```python
from build123d import *

# Parameters (mm, degrees)
SKETCH081_W      = 75
SKETCH081_H      = 95.5
EXTRUDE073_DEPTH = 1
SKETCH071_W      = 85
SKETCH071_H      = 109.5
EXTRUDE061_DEPTH = 2


with BuildPart() as extrude073:
    # Sketch081 → Extrude073 (new body)
    with BuildSketch(Plane.XY.offset(4)):
        with Locations((37.5, 49.25)):
            Rectangle(SKETCH081_W, SKETCH081_H)
    extrude(amount=EXTRUDE073_DEPTH)


with BuildPart() as cut008:
    # Sketch071 → Extrude061 (new body)
    with BuildSketch(Plane.XY.offset(3)):
        with Locations((37.5, 51.25)):
            Rectangle(SKETCH071_W, SKETCH071_H)
    extrude(amount=EXTRUDE061_DEPTH)

    # Cut008: cut Extrude073
    add(extrude073.part, mode=Mode.SUBTRACT)


solid = cut008.part
```
Geometry: final body of the model. Coordinates: model frame, mm. Coordinates: 2 decimals unless noted, no trailing zeros. Order: outer loops, then holes, each group sorted by start corner. A loop starts at its lowest first (then second) coordinate and runs counter-clockwise, first axis right, second up. Notation, with made-up numbers: (65.25, 80.5) - (87.25, 80.5) arc R20 cw to (87.25, 91.5) - close; hole circle Ø10 at (38.5, -22). An arc over 180 degrees is marked (long way). Write each question's results on one line, items separated by ' | '.
(1) Section query A-A, the plane z = 4.65. Return the cut outline in (x, y), plus the area to 4 significant figures.
Values found:
outline: (-5, -3.5) - (80, -3.5) - (80, 106) - (-5, 106) - close; hole (0, 1.5) - (75, 1.5) - (75, 97) - (0, 97) - close | area: 2,145 mm²
(2) Mould query, pull axis X, two halves, no side actions, for faces 1 (the face through (37, 50, 4)), 2 (the face through (37, 52, 3)). Classes: +X half, -X half, draft (parallel to the pull), parting line (faces both ways), or undercut.
Values found:
face 1: undercut | face 2: draft
(3) First-contact query: pin 1 Ø5 at (x, y) = (30, 77) entering from +Z. Flat tip, straight axial feed; report the tip coordinate or a pass-through.
Values found:
pin 1: stops at z = 4
(4) Section query C-C, the plane y = 75.5. Return the cut outline in (x, z), plus the area to 3 significant figures.
Values found:
outline: (-5, 3) - (80, 3) - (80, 5) - (75, 5) - (75, 4) - (0, 4) - (0, 5) - (-5, 5) - close | area: 95.0 mm²
(5) Line query: line 1 (X direction, y = 71, z = 4.65); line 2 (Y direction, x = 12.5, z = 4.9); line 3 (Z direction, x = 18.5, y = 69). Output: solid intervals per line, ascending. Write a range as [from, to].
Values found:
line 1: x = [-5, 0], [75, 80] | line 2: y = [-3.5, 1.5], [97, 106] | line 3: z = [3, 4]
(6) Section query B-B, the plane x = 63. Return the cut outline in (y, z), plus the area to 4 significant figures.
Values found:
outline: (-3.5, 3) - (106, 3) - (106, 5) - (97, 5) - (97, 4) - (1.5, 4) - (1.5, 5) - (-3.5, 5) - close | area: 123.5 mm²
